```python
from build123d import *

# Parameters (mm, degrees)
SKETCH1_R                                      = 2.55
BOSS_EXTRUDE1_DEPTH                            = 3
SKETCH2_R                                      = 10.5
CUT_EXTRUDE2_DEPTH                             = 4
CSK_FOR_M3_FLAT_HEAD_MACHINE_SCREW1_AT_2_COUNT = 2
CSK_FOR_M3_FLAT_HEAD_MACHINE_SCREW1_AT_2_PITCH = 26.084685162
CSK_FOR_M3_FLAT_HEAD_MACHINE_SCREW1_AT_3_COUNT = 2
CSK_FOR_M3_FLAT_HEAD_MACHINE_SCREW1_AT_3_PITCH = 26.084685162


with BuildPart() as part:
    # Sketch1 → Boss-Extrude1 (new body)
    with BuildSketch(Plane(origin=(0, 0, 0), x_dir=(1, 0, 0), z_dir=(0, 1, 0))):
        with BuildLine():
            Line((14.75, -33.5), (-14.75, -33.5))
            ThreePointArc((-14.75, -33.5), (-18.285533906, -32.035533906), (-19.75, -28.5))
            Line((-19.75, -28.5), (-19.75, 28.5))
            ThreePointArc((-19.75, 28.5), (-18.285533906, 32.035533906), (-14.75, 33.5))
            Line((-14.75, 33.5), (14.75, 33.5))
            ThreePointArc((14.75, 33.5), (18.285533906, 32.035533906), (19.75, 28.5))
            Line((19.75, 28.5), (19.75, -28.5))
            ThreePointArc((19.75, -28.5), (18.285533906, -32.035533906), (14.75, -33.5))
        make_face()
        with Locations((0, 26.5)):
            Circle(SKETCH1_R, mode=Mode.SUBTRACT)
        with Locations((10, -25.29)):
            Circle(SKETCH1_R, mode=Mode.SUBTRACT)
        with Locations((10, -5.29)):
            Circle(SKETCH1_R, mode=Mode.SUBTRACT)
        with Locations((0, -25.29)):
            Circle(SKETCH1_R, mode=Mode.SUBTRACT)
        with Locations((0, -5.29)):
            Circle(SKETCH1_R, mode=Mode.SUBTRACT)
        with Locations((-10, -25.29)):
            Circle(SKETCH1_R, mode=Mode.SUBTRACT)
        with Locations((-10, -5.29)):
            Circle(SKETCH1_R, mode=Mode.SUBTRACT)
    extrude(amount=BOSS_EXTRUDE1_DEPTH)

    # Sketch2 → Cut-Extrude2 (cut, through all)
    with BuildSketch(Plane(origin=(0, 3, 0), x_dir=(1, 0, 0), z_dir=(0, 1, 0))):
        with Locations((0, 20)):
            Circle(SKETCH2_R)
    extrude(amount=-CUT_EXTRUDE2_DEPTH, mode=Mode.SUBTRACT)

    # Sketch4 → CSK for M3 Flat Head Machine Screw1 (revolve, cut)
    with BuildSketch(Plane(origin=(-13.042342581, 3, -27.53), x_dir=(0, 0, 1), z_dir=(1, 0, 0))):
        Polygon((0, 0), (0, 3), (1.8, 3), (1.8, 1.85), (3.65, 0), align=None)
    csk_for_m3_flat_head_machine_screw1 = revolve(axis=Axis((-13.042342581, 9.35, -27.53), (0, -1, 0)), mode=Mode.SUBTRACT)

    # CSK for M3 Flat Head Machine Screw1 at 2: CSK for M3 Flat Head Machine Screw1 ×2
    with Locations(*[(i * CSK_FOR_M3_FLAT_HEAD_MACHINE_SCREW1_AT_2_PITCH, 0, 0) for i in range(1, CSK_FOR_M3_FLAT_HEAD_MACHINE_SCREW1_AT_2_COUNT)]):
        add(csk_for_m3_flat_head_machine_screw1, mode=Mode.SUBTRACT)

    # CSK for M3 Flat Head Machine Screw1 at 3: CSK for M3 Flat Head Machine Screw1 ×2
    with Locations(*[Vector(0.5, 0, 0.866025404) * (i * CSK_FOR_M3_FLAT_HEAD_MACHINE_SCREW1_AT_3_PITCH) for i in range(1, CSK_FOR_M3_FLAT_HEAD_MACHINE_SCREW1_AT_3_COUNT)]):
        add(csk_for_m3_flat_head_machine_screw1, mode=Mode.SUBTRACT)


solid = part.part
```
CAD build for the part. Positions are in the model's coordinates, mm. Coordinates: 2 decimals unless noted, no trailing zeros. Loops run counter-clockwise (first coordinate to the right, second up) from the corner with the lowest first, then second, coordinate; pieces in that order, holes last. Notation, with made-up numbers: (1.25, -7) - (6.25, -7) arc R5 ccw to (6.25, -2) - close; hole circle Ø11 at (82, -32). An arc over 180 degrees is marked (long way). Return JSON: item names as keys, results as strings.
1. Drop a flat-ended pin along its axis: pin 1 (4.5 mm diameter, centred on x = 0, z = 5.29, fed in from +Y). Give the stop position or say it passes through.
Result:
{"pin 1": "passes through"}
2. Probe L1, parallel to X at y = 0.9, z = 5.29; L2, parallel to Z at x = 0, y = 0.5; L3, parallel to X at y = 1.5, z = -28. List the from-to ranges inside material, lowest first. Write a range as from..to.
Result:
{"L1": "x = -19.75..-12.55, -7.45..-2.55, 2.55..7.45, 12.55..19.75", "L2": "z = -33.5..-30.5, -9.5..-6.74, -3.14..2.74, 7.84..22.74, 27.84..33.5", "L3": "x = -19.75..-15.14, -10.94..-6.8, 6.8..10.94, 15.14..19.75"}
3. Mould opens along Z. For faces 1 (the flat face through (-19.75, 1, 0)), 2 (the cylindrical face through (-12.024, 1.479, 26.842)), 3 (the cylindrical face through (18.32, 1.48, 32)), 4 (the cylindrical face through (-10.33, 1.48, 2.76)) say: released by +Z, released by -Z, zero draft, split by the parting line, or undercut.
Result:
{"face 1": "zero draft", "face 2": "undercut", "face 3": "released by +Z", "face 4": "undercut"}
4. Band-saw the part on C-C (y = 1.7). State how many separate pieces and enclosed holes the cut face has, and give its area (3 significant figures).
Result:
{"separate pieces": "1", "enclosed holes": "10", "area": "2,100 mm2"}
5. Band-saw the part on A-A (z = 25.29). Give the cut face in (x, y), and give its area (3 significant figures).
Result:
{"outline": "(-19.75, 0) - (-12.55, 0) - (-12.55, 3) - (-19.75, 3) - close; (-7.45, 0) - (-2.55, 0) - (-2.55, 3) - (-7.45, 3) - close; (2.55, 0) - (7.45, 0) - (7.45, 3) - (2.55, 3) - close; (12.55, 0) - (19.75, 0) - (19.75, 3) - (12.55, 3) - close", "area": "72.6 mm2"}
6. Band-saw the part on B-B (z = -20). Give the cut face in (x, y).
Result:
{"outline": "(-19.75, 0) - (-10.5, 0) - (-10.5, 3) - (-19.75, 3) - close; (10.5, 0) - (19.75, 0) - (19.75, 3) - (10.5, 3) - close"}
